from build123d import *

# Parameters (mm, degrees)
SKETCH2_W            = 64
SKETCH2_H            = 16.26
BASE_FLANGE1_DEPTH   = 3
EDGE_FLANGE1_DEPTH   = 18
SKETCH10_R           = 2.5
CUT_EXTRUDE1_DEPTH   = 3
FILLET1_R            = 8
SKETCH14_R           = 2.5
SKETCH14_R_2         = 1
CUT_EXTRUDE5_DEPTH   = 3
SKETCH15_W           = 8
SKETCH15_H           = 10
TAB1_DEPTH           = 3
FILLET4_R            = 8
FILLET5_R            = 3
FILLET4_OF_MIRROR1_R = 8
FILLET5_OF_MIRROR1_R = 3


# Sheet-metal steps are written as plain solids
with BuildPart() as part:
    # Sketch2 → Base-Flange1 (new body)
    with BuildSketch(Plane.XY):
        Rectangle(SKETCH2_W, SKETCH2_H)
    extrude(amount=-BASE_FLANGE1_DEPTH)

    # Edge-Flange1 section (across the edge) → Edge-Flange1 (add)
    with BuildSketch(Plane(origin=(14, 8.8666, -3), x_dir=(0, -1, 0), z_dir=(1, 0, 0))):
        with BuildLine():
            Line((-3, 0.7366), (-3, 24))
            Line((-3, 24), (0, 24))
            Line((0, 24), (0, 0.7366))
            ThreePointArc((0, 0.7366), (0.215745145, 0.215745145), (0.7366, 0))
            Line((0.7366, 0), (0.7366, -3))
            ThreePointArc((0.7366, -3), (-1.905575199, -1.905575199), (-3, 0.7366))
        make_face()
    edge_flange1 = extrude(amount=EDGE_FLANGE1_DEPTH)

    # Sketch10 → Cut-Extrude1 (cut)
    with BuildSketch(Plane.XY):
        with Locations((-19, -0.13)):
            Circle(SKETCH10_R)
        with Locations((19, -0.13)):
            Circle(SKETCH10_R)
    extrude(amount=-CUT_EXTRUDE1_DEPTH, mode=Mode.SUBTRACT)

    # Fillet1
    fillet1_edges = [part.edges().sort_by_distance(p)[0] for p in [
        (32, -8.13, -1.5),
        (-32, -8.13, -1.5),
    ]]
    fillet(fillet1_edges, radius=FILLET1_R)

    # Sketch14 → Cut-Extrude5 (cut)
    with BuildSketch(Plane(origin=(0, 11.8666, 0), x_dir=(1, 0, 0), z_dir=(0, 1, 0))):
        with Locations(Location((23, 18.7366, 0), (0, 0, 270))):
            Circle(SKETCH14_R)
        with Locations((37, 22)):
            Circle(SKETCH14_R_2)
    cut_extrude5 = extrude(amount=-CUT_EXTRUDE5_DEPTH, mode=Mode.SUBTRACT)

    # Sketch15 → Tab1 (add)
    with BuildSketch(Plane(origin=(0, 11.8666, 0), x_dir=(1, 0, 0), z_dir=(0, 1, 0))):
        with Locations((36, 8.7366)):
            Rectangle(SKETCH15_W, SKETCH15_H)
    tab1 = extrude(amount=-TAB1_DEPTH)

    # Fillet4
    fillet4_edges = [part.edges().sort_by_distance(p)[0] for p in [
        (14, 10.3666, -27),
        (32, 10.3666, -27),
    ]]
    fillet(fillet4_edges, radius=FILLET4_R)

    # Fillet5
    fillet5_edges = [part.edges().sort_by_distance(p)[0] for p in [
        (32, 10.3666, -13.7366),
        (40, 10.3666, -13.7366),
        (40, 10.3666, -3.7366),
    ]]
    fillet(fillet5_edges, radius=FILLET5_R)

    # Mirror1: Edge-Flange1, Cut-Extrude5, Tab1 across plane
    add(edge_flange1.mirror(Plane(origin=(0, 0, 0), x_dir=(0, 0, 1), z_dir=(1, 0, 0))))
    add(cut_extrude5.mirror(Plane(origin=(0, 0, 0), x_dir=(0, 0, 1), z_dir=(1, 0, 0))), mode=Mode.SUBTRACT)
    add(tab1.mirror(Plane(origin=(0, 0, 0), x_dir=(0, 0, 1), z_dir=(1, 0, 0))))

    # Fillet4 of Mirror1
    fillet4_of_mirror1_edges = [part.edges().sort_by_distance(p)[0] for p in [
        (-14, 10.3666, -27),
        (-32, 10.3666, -27),
    ]]
    fillet(fillet4_of_mirror1_edges, radius=FILLET4_OF_MIRROR1_R)

    # Fillet5 of Mirror1
    fillet5_of_mirror1_edges = [part.edges().sort_by_distance(p)[0] for p in [
        (-32, 10.3666, -13.7366),
        (-40, 10.3666, -13.7366),
        (-40, 10.3666, -3.7366),
    ]]
    fillet(fillet5_of_mirror1_edges, radius=FILLET5_OF_MIRROR1_R)


solid = part.part
Source: CAD feature listing. Evaluate the final solid. Frame: model axes, mm. A direction names the side the tool comes from. Round coordinates to 2 decimals unless told otherwise and drop trailing zeros. Loops run counter-clockwise (first coordinate to the right, second up) from the corner with the lowest first, then second, coordinate; pieces in that order, holes last.
Q1. Access query for faces 5 (the face through (-24, 8.867, -13)), 6 (the face through (0, 8.13, -1)), 7 (the face through (32, 10, -18)). Directions: +Z, -Z, +X, -X, +Y, -Y. A direction counts if a zero-diameter tool reaches every point of the face in a straight line with its end or side. Return the directions, or none.
Q2. Section A-A, the plane x = 23. Return loops of the section in (y, z), plus the area to 3 significant figures.
Q3. Section D-D, the plane z = -24.75. Return loops of the section in (x, y).
Q4. Ray query, line 1 (Z direction, x = 4, y = 4); line 2 (Y direction, x = 26.5, z = -22.25); line 3 (X direction, y = 10.25, z = -4.25). Return the intervals inside material, ascending.
Q5. Mould query, pull axis X, two halves, no side actions, for faces 1 (the face through (36, 10, -13.737)), 2 (the face through (25.48, 10.39, -19.06)), 3 (the face through (16.281, 10.346, -24.594)), 4 (the face through (29.719, 10.346, -24.594)). Classes: pulls with the +X half, pulls with the -X half, needs draft (parallel to the pull), parting line crosses it, or undercut.
Q6. First-contact query: P1, Ø1.8, axis at y = 10, z = -18.5, coming from the -X side; P2, Ø0.6, axis at x = -36.5, y = 9.5, coming from the -Z side; P3, Ø7, axis at x = -27.5, z = -13, coming from the -Y side. Flat tips, straight axial feed; report the tip coordinate or a pass-through.
Q7. Section C-C, the plane x = -19. Return loops of the section in (y, z), plus the area to 3 significant figures.
Q8. Section B-B, the plane z = -8.75. Return loops of the section in (x, y).
Solutions:
1. face 5: -Z, +X, -X, -Y
1. face 6: +Z, -Z, +Y
1. face 7: -Z, +X, +Y, -Y
2. outline: (-8.13, -3) - (8.13, -3) arc R0.74 cw to (8.87, -3.74) - (8.87, -16.24) - (11.87, -16.24) - (11.87, -3.74) arc R3.74 ccw to (8.13, 0) - (-8.13, 0) - close; (8.87, -27) - (11.87, -27) - (11.87, -21.24) - (8.87, -21.24) - close
2. area: 114 mm2
3. outline: (-29.56, 8.87) - (-16.44, 8.87) - (-16.44, 11.87) - (-29.56, 11.87) - close; (16.44, 8.87) - (29.56, 8.87) - (29.56, 11.87) - (16.44, 11.87) - close
4. line 1: z = -3 to 0
4. line 2: y = 8.87 to 11.87
4. line 3: x = -38.68 to -14, 14 to 38.68
5. face 1: needs draft
5. face 2: undercut
5. face 3: undercut
5. face 4: pulls with the +X half
6. P1: stops at x = -32
6. P2: stops at z = -13.74
6. P3: stops at y = 8.87
7. outline: (-8.13, -3) - (-2.63, -3) - (-2.63, 0) - (-8.13, 0) - close; (2.37, -3) - (8.13, -3) arc R0.74 cw to (8.87, -3.74) - (8.87, -26.42) - (11.87, -26.42) - (11.87, -3.74) arc R3.74 ccw to (8.13, 0) - (2.37, 0) - close
7. area: 112 mm2
8. outline: (-40, 8.87) - (-14, 8.87) - (-14, 11.87) - (-40, 11.87) - close; (14, 8.87) - (40, 8.87) - (40, 11.87) - (14, 11.87) - close
